Autodesk Inventor part; units mm, degrees
ref_plane "Начальная плоскость" through (0, 0, 0) normal (0, 0, 1) x (1, 0, 0)
ref_plane "Конечная плоскость" through (0, 0, 110) normal (0, 0, 1) x (1, 0, 0)
ref_plane "YZ Plane" through (0, 0, 0) normal (1, 0, 0) x (0, 1, 0)
ref_plane "Начальная плоскость" through (0, 0, 0) normal (0, 0, 1) x (1, 0, 0)
ref_plane "Конечная плоскость" through (0, 0, 110) normal (0, 0, 1) x (1, 0, 0)
sketch "Эскиз" plane through (0, 0, 0) normal (0, 0, 1) x (1, 0, 0)
  line L0 (-25, -20.5) -> (-25, 20.5)
  line L1 (-20.5, 25) -> (20.5, 25)
  line L2 (25, 20.5) -> (25, -20.5)
  line L3 (20.5, -25) -> (-20.5, -25)
  arc A0 (-25, -20.5) -> (-20.5, -25) centre (-20.5, -20.5) ccw
  arc A1 (-20.5, 25) -> (-25, 20.5) centre (-20.5, 20.5) ccw
  arc A2 (25, 20.5) -> (20.5, 25) centre (20.5, 20.5) ccw
  arc A3 (20.5, -25) -> (25, -20.5) centre (20.5, -20.5) ccw
  arc A4 (-20.5, 22) -> (-22, 20.5) centre (-20.5, 20.5) ccw
  line L4 (-20.5, 22) -> (20.5, 22)
  arc A5 (22, 20.5) -> (20.5, 22) centre (20.5, 20.5) ccw
  line L5 (22, 20.5) -> (22, -20.5)
  arc A6 (20.5, -22) -> (22, -20.5) centre (20.5, -20.5) ccw
  line L6 (20.5, -22) -> (-20.5, -22)
  arc A7 (-22, -20.5) -> (-20.5, -22) centre (-20.5, -20.5) ccw
  line L7 (-22, -20.5) -> (-22, 20.5)
  line L8 (0, 37.1021) -> (0, -37.1021) construction
  line L9 (-23.1021, 0) -> (23.1021, 0) construction
  dimension "d7" = 4.5
  dimension "d10" = 50
  dimension "d11" = 50
  dimension "d12" = 3
  dimension "d15" = 25
  dimension "d16" = 25
extrude "Базовый элемент" add sketch "Эскиз" along normal up to surface (110 mm away) from surface at 0
sketch "Sketch3" plane through (0, 0, 0) normal (0, 0, 1) x (1, 0, 0)
  line L0 (0, 0) -> (10, 0)
ref_plane "Work Plane3" through (0, 0, 0) normal (0, -1, 0) x (1, 0, 0)
sketch "Sketch4" plane through (0, 0, 0) normal (0, -1, 0) x (1, 0, 0)
  line L0 (-2, 0) -> (12, 0)
  line L1 (-2, 110) -> (12, 110)
  dimension "d18" = 110
sketch "Эскиз5" plane through (-20.5, -25, 110) normal (0, 0, 1) x (1, 0, 0)
  line L0 (-1.5, 45.5) -> (-1.5, 4.5)
  line L1 (41, 47) -> (0, 47)
  line L2 (41, 47) -> (0, 47)
  arc A0 (42.5, 45.5) -> (41, 47) centre (41, 45.5) ccw
  line L3 (42.5, 4.5) -> (42.5, 45.5)
  arc A1 (41, 3) -> (42.5, 4.5) centre (41, 4.5) ccw
  line L4 (0, 3) -> (41, 3)
  arc A2 (-1.5, 4.5) -> (0, 3) centre (0, 4.5) ccw
  line L5 (-1.5, 45.5) -> (-1.5, 4.5)
  arc A3 (0, 47) -> (-1.5, 45.5) centre (0, 45.5) ccw
  line L6 (-4.5, 4.5) -> (-4.5, 45.5)
  arc A4 (-4.5, 4.5) -> (0, 0) centre (0, 4.5) ccw
  line L7 (41, 0) -> (0, 0)
  arc A5 (41, 0) -> (45.5, 4.5) centre (41, 4.5) ccw
  line L8 (45.5, 45.5) -> (45.5, 4.5)
  arc A6 (45.5, 45.5) -> (41, 50) centre (41, 45.5) ccw
  line L9 (0, 50) -> (41, 50)
  arc A7 (0, 50) -> (-4.5, 45.5) centre (0, 45.5) ccw
  point P0 (20.5, 25)
  point P1 (0, 47)
extrude "Выдавливание2" add sketch "Эскиз5" along normal blind 14
sketch "Эскиз6" plane through (-20.5, -25, 124) normal (0, 0, 1) x (1, 0, 0)
  line L0 (45.5, 4.5) -> (45.5, 45.5)
  arc A0 (45.5, 45.5) -> (41, 50) centre (41, 45.5) ccw
  line L1 (41, 50) -> (0, 50)
  arc A1 (0, 50) -> (-4.5, 45.5) centre (0, 45.5) ccw
  line L2 (-4.5, 45.5) -> (-4.5, 4.5)
  arc A2 (-4.5, 4.5) -> (0, 0) centre (0, 4.5) ccw
  line L3 (0, 0) -> (41, 0)
  arc A3 (41, 0) -> (45.5, 4.5) centre (41, 4.5) ccw
  arc A4 (42.5, 45.5) -> (41, 47) centre (41, 45.5) ccw
  line L4 (42.5, 45.5) -> (42.5, 4.5)
  arc A5 (41, 3) -> (42.5, 4.5) centre (41, 4.5) ccw
  line L5 (41, 3) -> (0, 3)
  arc A6 (-1.5, 4.5) -> (0, 3) centre (0, 4.5) ccw
  line L6 (-1.5, 4.5) -> (-1.5, 45.5)
  arc A7 (0, 47) -> (-1.5, 45.5) centre (0, 45.5) ccw
  line L7 (0, 47) -> (41, 47)
  line L8 (0, 49) -> (41, 49)
  arc A8 (44.5, 45.5) -> (41, 49) centre (41, 45.5) ccw
  line L9 (44.5, 45.5) -> (44.5, 4.5)
  arc A9 (41, 1) -> (44.5, 4.5) centre (41, 4.5) ccw
  line L10 (41, 1) -> (0, 1)
  arc A10 (-3.5, 4.5) -> (0, 1) centre (0, 4.5) ccw
  line L11 (-3.5, 4.5) -> (-3.5, 45.5)
  arc A11 (0, 49) -> (-3.5, 45.5) centre (0, 45.5) ccw
  point P0 (20.5, 25)
  dimension "d21" = 3
  dimension "d22" = 1
extrude "Выдавливание3" cut sketch "Эскиз6" against normal blind 150.25 contours A3 L3 A2 L2 A1 L1 A0 L0
equation "\"d7\" = G_IR"
equation "\"d10\" = G_H"
equation "\"d11\" = G_W"
equation "\"d12\" = G_T"
equation "\"d15\" = 0.5 * d10"
equation "\"d16\" = 0.5 * d11"
equation "\"d3\" = G_L"
equation "\"G_W\" = 50"
equation "\"G_H\" = 50"
equation "\"G_T\" = 3"
equation "\"G_IR\" = 1.5 * G_T"
equation "\"G_L\" = d18"
equation "\"G_OFFSET_START\" = 0"
equation "\"G_OFFSET_END\" = 0"
properties part number "Труба 50x50x3 -110 ГОСТ 8639-82" material "Сталь нержавеющая AISI 202"
Geometry: final body of the model. Coordinates: model frame, mm. A direction names the side the tool comes from. Coordinates: 2 decimals unless noted, no trailing zeros. Order: outer loops, then holes, each group sorted by start corner. A loop starts at its lowest first (then second) coordinate and runs counter-clockwise, first axis right, second up.
1) Section A-A (x = -10.5). Return loops of the section in (y, z), then the cut area to 3 significant figures.
Result sheet:
outline: (-24, 0) - (-22, 0) - (-22, 124) - (-24, 124) - close; (22, 0) - (24, 0) - (24, 124) - (22, 124) - close
area: 496 mm2
2) Section C-C (z = 80.5). Return loops of the section in (x, y), then the cut area to 3 significant figures.
Result sheet:
outline: (-24, -20.5) arc R3.5 ccw to (-20.5, -24) - (20.5, -24) arc R3.5 ccw to (24, -20.5) - (24, 20.5) arc R3.5 ccw to (20.5, 24) - (-20.5, 24) arc R3.5 ccw to (-24, 20.5) - close; hole (-22, -20.5) arc R1.5 ccw to (-20.5, -22) - (20.5, -22) arc R1.5 ccw to (22, -20.5) - (22, 20.5) arc R1.5 ccw to (20.5, 22) - (-20.5, 22) arc R1.5 ccw to (-22, 20.5) - close
area: 359 mm2
3) Set-up query: faces 5 (the flat face through (0, 24, 63)), 6 (the flat face through (0, 22, 61)). Return all of +Z, -Z, +X, -X, +Y, -Y with unobstructed straight access to the full face (end or side cutting, diameter ignored); none if empty.
Result sheet:
face 5: +Z, -Z, +X, -X, +Y
face 6: +Z, -Z
4) Draft query along X for faces 1 (the flat face through (0, -24, 63)), 2 (the flat face through (-22, 0, 61)), 3 (the cylindrical face through (23, 22.95, 62.87)), 4 (the cylindrical face through (-23, -22.95, 62.87)). Return one class per face: released by +X, released by -X, zero draft, split by the parting line, or undercut.
Result sheet:
face 1: zero draft
face 2: undercut
face 3: released by +X
face 4: released by -X
5) Ray query, probe 1 along Y at (x, z) = (-20, 81); probe 2 along Y at (x, z) = (-21, 87). Return the intervals inside material, ascending.
Result sheet:
probe 1: y = -24 to -22, 22 to 24
probe 2: y = -23.96 to -21.91, 21.91 to 23.96
